Design review of the part built by this model. Coordinates are the model's own, in mm. Coordinates: 2 decimals unless noted, no trailing zeros. Write each loop counter-clockwise with the first axis right and the second up, starting at its lowest first coordinate (ties: lowest second). Pieces come first, ordered by that corner, then holes. Notation, with made-up numbers: (38, -27) - (86, -27) arc R25 cw to (86, 5) - close; hole circle Ø7 at (-37.5, 55). An arc over 180 degrees is marked (long way). Use a Markdown table: item, result.
from build123d import *

# Parameters (mm, degrees)
BOSS_EXTRU_1_DEPTH   = 3
D_GAGEMENT_M41_D     = 4.4
D_GAGEMENT_M41_DEPTH = 5


with BuildPart() as part:
    # Esquisse4 → Boss.-Extru.1 (new body)
    with BuildSketch(Plane(origin=(0, 0, 0), x_dir=(1, 0, 0), z_dir=(0, 1, 0))):
        Polygon((197.809683941, 105.737894452), (157.80968394, 129.737894452), (157.80968394, 149.737894452), (65.80968453, 149.737894452), (65.80968453, 105.737894452), (-74.19031547, 105.737894452), (-74.19031547, 149.737894452), (-162.1903155, 149.737894452), (-162.1903155, 105.737894452), (-222.1903155, 105.737894452), (-222.1903155, -106.262104989), (-162.1903155, -106.262104989), (-162.1903155, -150.262104989), (-74.19031547, -150.262104989), (-74.19031547, -106.262104989), (65.80968453, -106.262104989), (65.80968453, -150.262104989), (157.80968394, -150.262104989), (157.80968394, -130.262104989), (197.809683941, -106.262104989), (217.809683941, -106.262104989), (217.809683941, 105.737894452), align=None)
    extrude(amount=BOSS_EXTRU_1_DEPTH)

    # Dégagement M41
    with Locations(Plane(origin=(0, 0, 0), x_dir=(-1, 0, 0), z_dir=(0, -1, 0))):
        with Locations((-207.809683941, 85.737894452), (-207.809683941, -86.262104989), (-111.809684235, -140.262104989), (118.190315485, -140.262104989), (-111.809684235, 139.737894452), (118.190315485, 139.737894452), (212.1903155, 85.737894452), (212.1903155, -86.262104989)):
            Hole(D_GAGEMENT_M41_D / 2, depth=D_GAGEMENT_M41_DEPTH)


solid = part.part
(1) Take a section at A-A on y = 1.65. State how many separate pieces and enclosed holes the cut face has, and give its area (3 significant figures).
Determined:
| item | result |
|---|---|
| separate pieces | 1 |
| enclosed holes | 8 |
| area | 110,000 mm2 |
(2) Take a section at B-B on x = -17. Write out the cut boundary in (y, z).
Determined:
| item | result |
|---|---|
| outline | (0, -105.74) - (3, -105.74) - (3, 106.26) - (0, 106.26) - close |
(3) For pin 1 (0.9 mm diameter, centred on y = 2, z = -129, fed in from +X); pin 2 (0.9 mm diameter, centred on y = 1, z = 134, fed in from -X); pin 3 (4 mm diameter, centred on x = -118.19, z = 140.26, fed in from +Y); pin 4 (1.5 mm diameter, centred on y = 1, z = 129.5, fed in from +X), all flat-tipped, find the tip position at first contact; note any pin that passes through.
Determined:
| item | result |
|---|---|
| pin 1 | x = 159.79 |
| pin 2 | x = -162.19 |
| pin 3 | through |
| pin 4 | x = 160.33 |
(4) Take a section at C-C on x = 180.5. Write out the cut boundary in (y, z), and give its area (3 significant figures).
Determined:
| item | result |
|---|---|
| outline | (0, -116.12) - (3, -116.12) - (3, 116.65) - (0, 116.65) - close |
| area | 698 mm2 |
(5) For L1, parallel to X at y = 2.7, z = 133.5; L2, parallel to Z at x = -200, y = 0.7; L3, parallel to X at y = 2.3, z = 114, list the stretches that pass through material, from the lowest coordinate up. Write a range as from..to.
Determined:
| item | result |
|---|---|
| L1 | -162.19..-74.19, 65.81..157.81 |
| L2 | -105.74..106.26 |
| L3 | -162.19..-74.19, 65.81..184.91 |
